Geometry check sheet. Reference: the model listing, model coordinates, mm. A direction names the side the tool comes from. Round coordinates to 2 decimals unless told otherwise and drop trailing zeros. Loops run counter-clockwise (first coordinate to the right, second up) from the corner with the lowest first, then second, coordinate; pieces in that order, holes last. Notation, with made-up numbers: (77.5, 35) -> (100.5, 35) arc R31 cw to (100.5, 73) -> close; hole circle Ø2 at (5, -2.75). An arc over 180 degrees is marked (long way). Use a Markdown table: item, result. Add a question column.
Q1. Release check for a two-part mould opening along X. For faces 1 (the face through (21.2, -14, -6)), 2 (the face through (66.172, 10.648, 13.887)), 3 (the face through (0, 0, 0)) record: released by +X, released by -X, zero draft, split by the parting line, or undercut.
Q2. Sectioned sample at D-D, the plane x = 39. Enter the section's corners in (y, z), then the cut area to 3 significant figures.
Q3. Set-up check for faces 4 (the face through (21, -0.1, 15.2)), 5 (the face through (64.2, -17, -6)), 6 (the face through (-6, -1, 4)), 7 (the face through (-21.5, 0, 7)), 8 (the face through (5, 0, 18)): record each of +Z, -Z, +X, -X, +Y, -Y from which the full face is reachable in a straight line by a thin tool's end or side.
Q4. Gauge pin test, flat ends, axial feed: P1, Ø5, axis at x = 57.5, z = 12, coming from the +Y side; P2, Ø1.5, axis at x = 40, y = 3.5, coming from the -Z side; P3, Ø12, axis at x = 31.5, z = 6, coming from the -Y side. Record the tip position at first contact, or that the pin passes through.
Q5. Material ranges on L1, parallel to X at y = -7, z = 5; L2, parallel to Y at x = 59.5, z = -0.5; L3, parallel to X at y = -1, z = 4, recorded low to high.
Q6. Sectioned sample at A-A, the plane z = 0. Enter the section's corners in (x, y).
Q7. Sectioned sample at C-C, the plane x = 8. Enter the section's corners in (y, z).
Autodesk Inventor part; units mm, degrees
ref_plane "YZ Plane" through (0, 0, 0) normal (1, 0, 0) x (0, 1, 0)
ref_plane "XZ Plane" through (0, 0, 0) normal (0, 1, 0) x (-1, 0, 0)
ref_plane "XY Plane" through (0, 0, 0) normal (0, 0, 1) x (1, 0, 0)
sketch "Эскиз1" plane through (0, 0, 0) normal (1, 0, 0) x (0, 1, 0)
  circle A0 centre (0, 0) radius 18.5
  dimension "d0" = 37
extrude "Выдавливание1" add sketch "Эскиз1" along normal blind 21
sketch "Эскиз2" plane through (21, 0, 0) normal (1, 0, 0) x (0, 0, -1)
  circle A0 centre (0, 0) radius 15
  dimension "d3" = 30
extrude "Выдавливание2" add sketch "Эскиз2" along normal blind 0.2
sketch "Эскиз3" plane through (21.2, 0, 0) normal (1, 0, 0) x (0, 0, -1)
  circle A0 centre (0, 0) radius 19
  dimension "d6" = 38
extrude "Выдавливание3" add sketch "Эскиз3" along normal blind 43
fillet "Сопряжение1" radius 2 1 edges at (21.2, 0, 19)
sketch "Эскиз4" plane through (64.2, 0, 0) normal (1, 0, 0) x (0, 0, -1)
  circle A0 centre (0, 0) radius 17.5
  dimension "d10" = 35
extrude "Выдавливание4" add sketch "Эскиз4" along normal blind 5
fillet "Сопряжение2" radius 1 1 edges at (69.2, 0, 17.5)
sketch "Эскиз5" plane through (0, 0, 0) normal (-1, 0, 0) x (0, 0, 1)
  line L0 (0, 0) -> (27.1698, 0) construction
  circle A0 centre (7, 0) radius 6
  dimension "d14" = 12
  dimension "d15" = 7
extrude "Выдавливание5" add sketch "Эскиз5" along normal blind 6
sketch "Эскиз6" plane through (-6, 0, 7) normal (-1, 0, 0) x (0, 0, 1)
  circle A0 centre (0, 0) radius 3
  circle A1 centre (0, 0) radius 6
  point P0 (-7, 0)
  dimension "d18" = 6
extrude "Выдавливание6" add sketch "Эскиз6" along normal blind 15.5 contours A0
sketch "Эскиз7" plane through (0, 0, 0) normal (-1, 0, 0) x (0, 0, 1)
  circle A0 centre (7, 0) radius 3
  line L0 (0, 0) -> (22.9048, 0) construction
  line L1 (21, 1) -> (18, 1)
  line L2 (18, 1) -> (18, -1)
  line L3 (18, -1) -> (21, -1)
  line L4 (21, -1) -> (21, 1)
  dimension "d21" = 18
  dimension "d22" = 3
  dimension "d23" = 2
extrude "Выдавливание7" cut sketch "Эскиз7" against normal blind 10 contours L4 L3 L2 L1
properties part number "Двигатель"
Values:
| question | item | result |
|---|---|---|
| 1 | face 1 | undercut |
| 1 | face 2 | zero draft |
| 1 | face 3 | released by -X |
| 2 | outline | circle Ø38 at (0, 0) |
| 2 | area | 1,130 mm^2 |
| 3 | face 4 | none |
| 3 | face 5 | +X |
| 3 | face 6 | -X |
| 3 | face 7 | +Z, -Z, -X, +Y, -Y |
| 3 | face 8 | +Z, -X |
| 4 | P1 | y = 16.45 |
| 4 | P2 | z = -18.8 |
| 4 | P3 | y = -19 |
| 5 | L1 | 0 to 69.2 |
| 5 | L2 | -18.99 to 18.99 |
| 5 | L3 | -6 to 69.2 |
| 6 | outline | (0, -18.5) -> (21, -18.5) -> (21, -15) -> (21.2, -15) -> (21.2, -17) arc R2 ccw to (23.2, -19) -> (64.2, -19) -> (64.2, -17.5) -> (68.2, -17.5) arc R1 ccw to (69.2, -16.5) -> (69.2, 16.5) arc R1 ccw to (68.2, 17.5) -> (64.2, 17.5) -> (64.2, 19) -> (23.2, 19) arc R2 ccw to (21.2, 17) -> (21.2, 15) -> (21, 15) -> (21, 18.5) -> (0, 18.5) -> close |
| 7 | outline | (-1, 18) -> (-1, 18.47) arc R18.5 ccw (long way) to (1, 18.47) -> (1, 18) -> close |
